Source: three-view drawing plus pictorial views. Frame: mm from the lowest corner of the part. Round coordinates to 2 decimals unless told otherwise and drop trailing zeros. Order: outer loops, then holes, each group sorted by start corner. A loop starts at its lowest first (then second) coordinate and runs counter-clockwise, first axis right, second up. Notation, with made-up numbers: (-2, 49) -> (16, 49) arc R20 ccw to (16, 67) -> close; hole circle Ø8 at (81, -2). An arc over 180 degrees is marked (long way). Use a Markdown table: item, result.
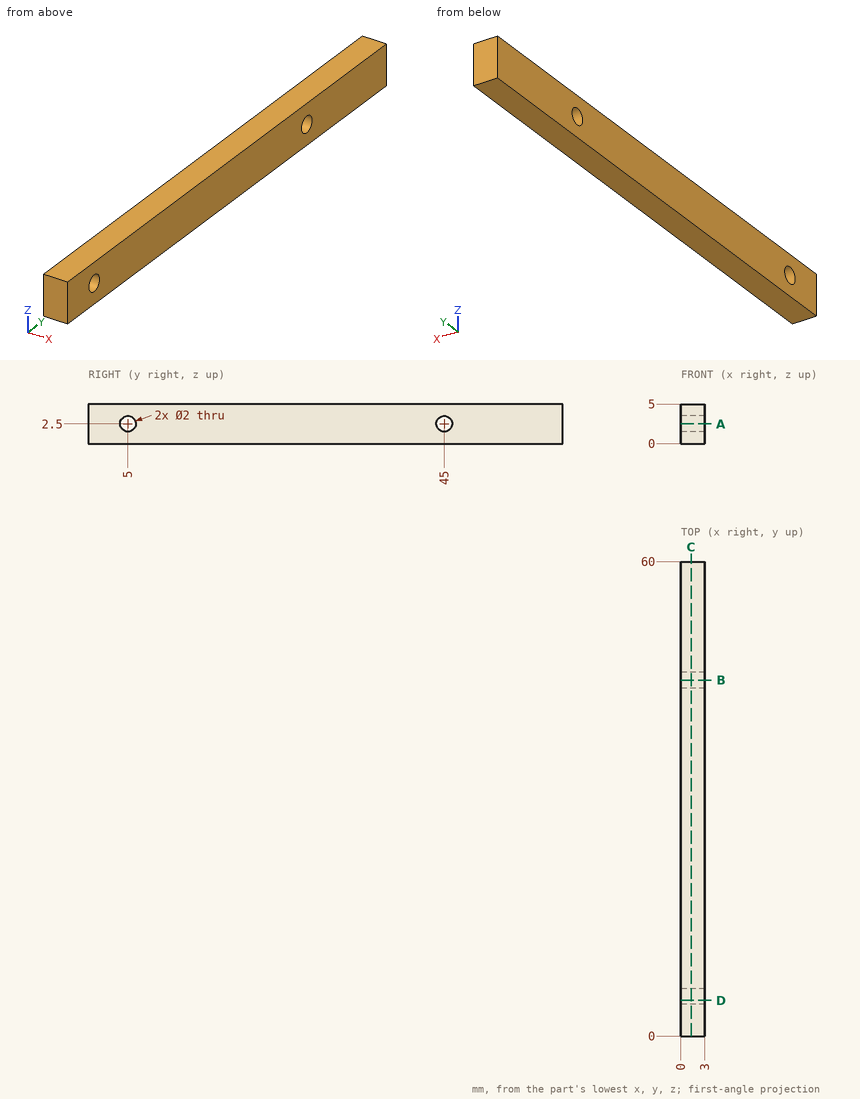
1) Pin query (flat end, axial travel): pin 1 Ø1.8 at (y, z) = (5, 2.5) entering from -X. Return the tip coordinate at first contact, or that it passes through.
Results found:
| item | result |
|---|---|
| pin 1 | passes through |
2) Cut plane C-C on x = 1.3. Return loops of the section in (y, z), and give its area (3 significant figures).
Results found:
| item | result |
|---|---|
| outline | (0, 0) -> (60, 0) -> (60, 5) -> (0, 5) -> close; hole circle Ø2 at (5, 2.5); hole circle Ø2 at (45, 2.5) |
| area | 294 mm² |
3) Line query: L1, parallel to Y at x = 1.75, z = 2.5; L2, parallel to Y at x = 1.65, z = 1.95; L3, parallel to Z at x = 0.85, y = 5. Output: solid intervals per line, ascending. Write a range as [from, to].
Results found:
| item | result |
|---|---|
| L1 | y = [0, 4], [6, 44], [46, 60] |
| L2 | y = [0, 4.16], [5.84, 44.16], [45.84, 60] |
| L3 | z = [0, 1.5], [3.5, 5] |
4) Cut plane D-D on y = 4.5. Return loops of the section in (x, z).
Results found:
| item | result |
|---|---|
| outline | (0, 0) -> (3, 0) -> (3, 1.63) -> (0, 1.63) -> close; (0, 3.37) -> (3, 3.37) -> (3, 5) -> (0, 5) -> close |
5) Cut plane B-B on y = 45. Return loops of the section in (x, z).
Results found:
| item | result |
|---|---|
| outline | (0, 0) -> (3, 0) -> (3, 1.5) -> (0, 1.5) -> close; (0, 3.5) -> (3, 3.5) -> (3, 5) -> (0, 5) -> close |
6) Cut plane A-A on z = 2.5. Return loops of the section in (x, y).
Results found:
| item | result |
|---|---|
| outline | (0, 0) -> (3, 0) -> (3, 4) -> (0, 4) -> close; (0, 6) -> (3, 6) -> (3, 44) -> (0, 44) -> close; (0, 46) -> (3, 46) -> (3, 60) -> (0, 60) -> close |
